For this review, use the dimensioned drawing (mm, ordinates from the lowest corner) and the shaded views. A direction names the side the tool comes from. Coordinates: 2 decimals unless noted, no trailing zeros. Loops run counter-clockwise (first coordinate to the right, second up) from the corner with the lowest first, then second, coordinate; pieces in that order, holes last.
1. Take a section at D-D, the plane z = 5. State the section outline as (x, y) points.
2. Machinability: for the marked faces 4, 5, 6, 7 and 8, which of the approach directions +Z, -Z, +X, -X, +Y, -Y give a long, thin tool a straight path to every point of the face, cutting with its end or side? Answer none if there is none.
3. Take a section at A-A, the plane z = 12. State the section outline as (x, y) points, then the cut area to 3 significant figures.
4. Take a section at B-B, the plane x = 10. State the section outline as (y, z) points, then the cut area to 3 significant figures.
5. To check wall thickness, follow probe 1 along Y at (x, z) = (9, 11.5); probe 2 along Z at (x, y) = (12.75, 7.25); probe 3 along X at (y, z) = (8, 13). State the ranges of each line that lie inside material, in increasing order.
6. Clearance check with flat-ended pins moving along their axes: P1, Ø6, axis at x = 15, z = 2.5, coming from the +Y side; P2, Ø1.8, axis at y = 9, z = 12.5, coming from the +X side; P3, Ø5, axis at x = 8.5, y = 14.5, coming from the +Z side. State where each tip first meets the part, or that it passes through.
7. Take a section at C-C, the plane z = 7. State the section outline as (x, y) points.
8. Mouldability with a two-part tool opening along Z and no side actions: class the marked faces 1, 2 and 3 as pulls with the +Z half, pulls with the -Z half, needs draft (parallel to the pull), parting line crosses it, or undercut.
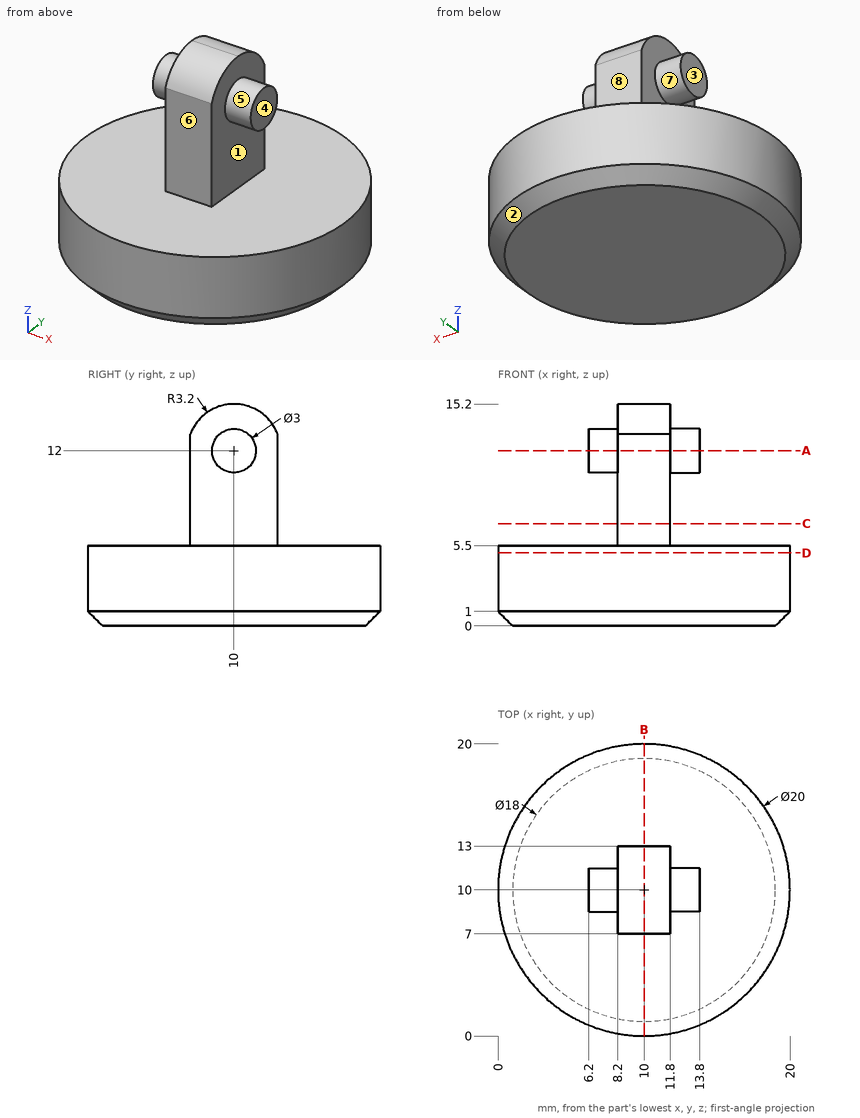
Results list:
1. outline: circle Ø20 at (10, 10)
2. face 4: +Z, +X, +Y, -Y
2. face 5: +X
2. face 6: +Z, +X, -X, -Y
2. face 7: -X
2. face 8: +Z, +X, -X, +Y
3. outline: (6.2, 8.5) - (8.2, 8.5) - (8.2, 7) - (11.8, 7) - (11.8, 8.5) - (13.8, 8.5) - (13.8, 11.5) - (11.8, 11.5) - (11.8, 13) - (8.2, 13) - (8.2, 11.5) - (6.2, 11.5) - close
3. area: 33.6 mm2
4. outline: (0, 1) - (1, 0) - (19, 0) - (20, 1) - (20, 5.5) - (13, 5.5) - (13, 13.11) arc R3.2 ccw to (7, 13.11) - (7, 5.5) - (0, 5.5) - close
4. area: 164 mm2
5. probe 1: y = 7 to 13
5. probe 2: z = 0 to 5.5
5. probe 3: x = 8.2 to 11.8
6. P1: stops at y = 19.8
6. P2: stops at x = 13.8
6. P3: stops at z = 14.5
7. outline: (8.2, 7) - (11.8, 7) - (11.8, 13) - (8.2, 13) - close
8. face 1: undercut
8. face 2: pulls with the -Z half
8. face 3: needs draft
